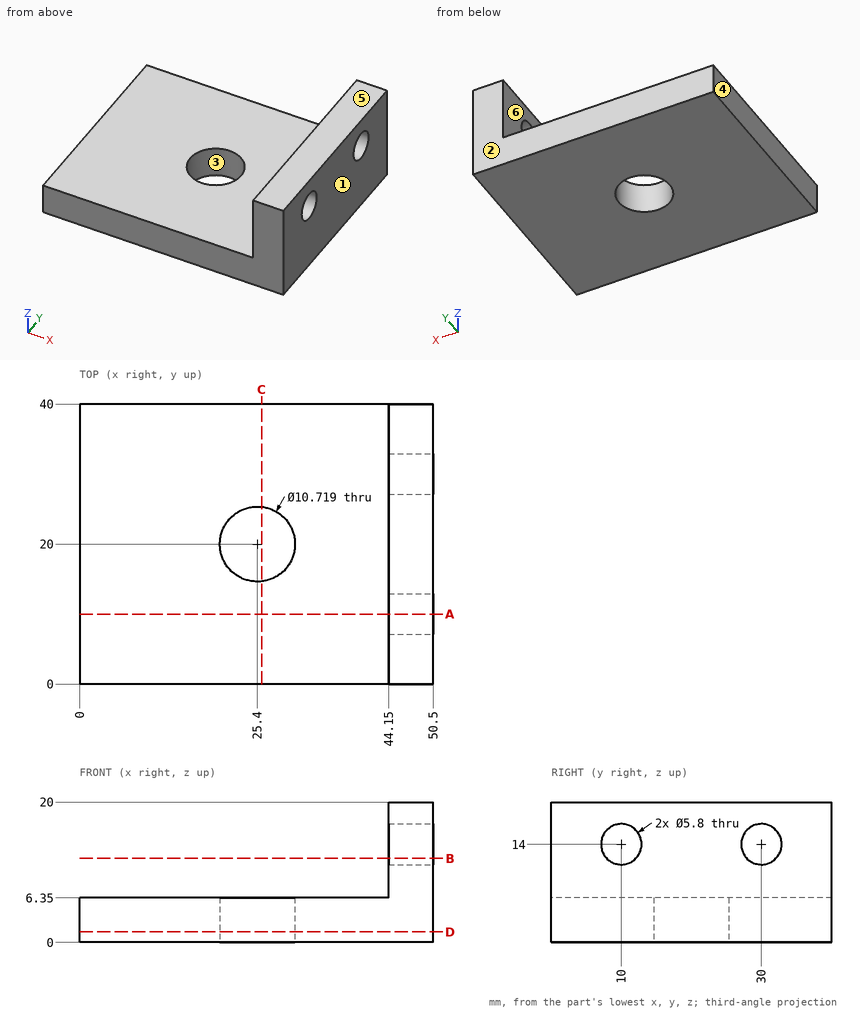
Drawing for the job (mm, zero at the part's lowest x, y, z). A direction names the side the tool comes from. Give positions to 0.01 mm unless a question says otherwise; leave off trailing zeros. Loops run counter-clockwise (first coordinate to the right, second up) from the corner with the lowest first, then second, coordinate; pieces in that order, holes last.
(1) Band-saw the part on A-A (y = 10). Write the cut outline in (x, z).
Return value:
outline: (0, 0) - (50.5, 0) - (50.5, 11.1) - (44.15, 11.1) - (44.15, 6.35) - (0, 6.35) - close; (44.15, 16.9) - (50.5, 16.9) - (50.5, 20) - (44.15, 20) - close
(2) 3-axis set-ups, long thin cutter, end or side, ignore diameter. For the marked faces 5 and 6: which of +Z, -Z, +X, -X, +Y, -Y reach the whole face in a straight line?
Return value:
face 5: +Z, +X, -X, +Y, -Y
face 6: +Z, -X, +Y, -Y
(3) Band-saw the part on D-D (z = 1.5). Write the cut outline in (x, y).
Return value:
outline: (0, 0) - (50.5, 0) - (50.5, 40) - (0, 40) - close; hole circle Ø10.72 at (25.4, 20)
(4) Band-saw the part on C-C (x = 26). Write the cut outline in (y, z), and give its area (3 significant figures).
Return value:
outline: (0, 0) - (14.67, 0) - (14.67, 6.35) - (0, 6.35) - close; (25.33, 0) - (40, 0) - (40, 6.35) - (25.33, 6.35) - close
area: 186 mm2
(5) Pin check, flat tip, straight feed: pin 1 (2 mm diameter, centred on x = 38, y = 25, fed in from +Z). Stop position of the tip, or through.
Return value:
pin 1: stops at z = 6.35
(6) Drill centre lines: line 1 along Y through (x, z) = (46, 14); line 2 along Z through (x, y) = (46, 30); line 3 along Y through (x, z) = (25.4, 4.25). Where is each one in solid material? Low to high.
Return value:
line 1: y = 0 to 7.1, 12.9 to 27.1, 32.9 to 40
line 2: z = 0 to 11.1, 16.9 to 20
line 3: y = 0 to 14.64, 25.36 to 40
(7) Pull direction X, two halves, no side cores. Call the marked faces 1, 2, 3 and 4: pulls with the +X half, pulls with the -X half, needs draft (parallel to the pull), parting line crosses it, or undercut.
Return value:
face 1: pulls with the +X half
face 2: needs draft
face 3: undercut
face 4: pulls with the -X half
(8) Band-saw the part on B-B (z = 12). Write the cut outline in (x, y), and give its area (3 significant figures).
Return value:
outline: (44.15, 0) - (50.5, 0) - (50.5, 7.9) - (44.15, 7.9) - close; (44.15, 12.1) - (50.5, 12.1) - (50.5, 27.9) - (44.15, 27.9) - close; (44.15, 32.1) - (50.5, 32.1) - (50.5, 40) - (44.15, 40) - close
area: 201 mm2
